Design review of the part built by this model. Coordinates are the model's own, in mm. A direction names the side the tool comes from. Round coordinates to 2 decimals unless told otherwise and drop trailing zeros. Order: outer loops, then holes, each group sorted by start corner. A loop starts at its lowest first (then second) coordinate and runs counter-clockwise, first axis right, second up.
from build123d import *

# Parameters (mm, degrees)
BOSS_EXTRUDE1_DEPTH = 222.25
SKETCH19_W          = 107.95
SKETCH19_H          = 139.7
BOSS_EXTRUDE2_DEPTH = 3.175


with BuildPart() as part:
    # Sketch18 → Boss-Extrude1 (new, symmetric)
    with BuildSketch(Plane(origin=(0, 0, 0), x_dir=(1, 0, 0), z_dir=(0, 1, 0))):
        Polygon((3.175, 38.1), (3.175, 3.175), (38.1, 3.175), (38.1, 0), (0, 0), (0, 38.1), align=None)
    extrude(amount=BOSS_EXTRUDE1_DEPTH, both=True)

    # Sketch19 → Boss-Extrude2 (add)
    with BuildSketch(Plane(origin=(0, 0, 0), x_dir=(0, 0, -1), z_dir=(1, 0, 0))):
        with Locations((92.075, -152.4)):
            Rectangle(SKETCH19_W, SKETCH19_H)
    extrude(amount=BOSS_EXTRUDE2_DEPTH)


solid = part.part
1) Clearance check with flat-ended pins moving along their axes: P1, Ø2.5, axis at x = 1.5, z = -71, coming from the +Y side; P2, Ø3, axis at x = 17, y = 36.5, coming from the -Z side (3 decimals); P3, Ø12, axis at y = 17.5, z = -22, coming from the +X side (3 decimals). State where each tip first meets the part, or that it passes through.
Results:
P1: stops at y = -82.55
P2: stops at z = -3.175
P3: stops at x = 3.175
2) Take a section at C-C on x = 17. Give the boundary of the cut face in (y, z) (3 decimals).
Results:
outline: (-222.25, -3.175) - (222.25, -3.175) - (222.25, 0) - (-222.25, 0) - close
3) Take a section at A-A on y = -96. Give the boundary of the cut face in (x, z) (3 decimals), plus the area to 3 significant figures.
Results:
outline: (0, -146.05) - (3.175, -146.05) - (3.175, -3.175) - (38.1, -3.175) - (38.1, 0) - (0, 0) - close
area: 575 mm2
4) To check wall thickness, follow line 1 along Z through (x, y) = (27, -45.5) (3 decimals); line 2 along X through (y, z) = (196, -35.5) (3 decimals). State the ranges of each line that lie inside material, in increasing order.
Results:
line 1: z = -3.175 to 0
line 2: x = 0 to 3.175
5) For faces 1 (the face through (11, 222.25, -2)), 2 (the face through (20, 3, -3.175)), list the 3-axis set-ups (+Z, -Z, +X, -X, +Y, -Y) from which the entire face can be reached by the end or side of a thin tool; tool diameter is ignored.
Results:
face 1: +Z, -Z, +X, -X, +Y
face 2: -Z, +X, +Y, -Y
6) Take a section at B-B on z = -87. Give the boundary of the cut face in (x, y) (3 decimals).
Results:
outline: (0, -222.25) - (3.175, -222.25) - (3.175, -82.55) - (0, -82.55) - close
